```python
from build123d import *

# Parameters (mm, degrees)
SKETCH1_W           = 25
SKETCH1_H           = 0.7
BOSS_EXTRUDE1_DEPTH = 40
SKETCH2_R           = 2.15
SKETCH2_R_2         = 1.5
CUT_EXTRUDE1_DEPTH  = 40


with BuildPart() as part:
    # Sketch1 → Boss-Extrude1 (new body)
    with BuildSketch(Plane(origin=(0, 0, 0), x_dir=(1, 0, 0), z_dir=(0, 1, 0))):
        with Locations((12.5, 0.35)):
            Rectangle(SKETCH1_W, SKETCH1_H)
    extrude(amount=BOSS_EXTRUDE1_DEPTH)

    # Sketch2 → Cut-Extrude1 (cut)
    with BuildSketch(Plane.XY):
        with Locations((4, 35)):
            Circle(SKETCH2_R)
        with Locations((4, 25)):
            Circle(SKETCH2_R)
        with Locations((4, 15)):
            Circle(SKETCH2_R_2)
        with Locations((4, 5)):
            Circle(SKETCH2_R_2)
        with Locations((19, 15)):
            Circle(SKETCH2_R_2)
        with Locations((19, 5)):
            Circle(SKETCH2_R_2)
    extrude(amount=-CUT_EXTRUDE1_DEPTH, mode=Mode.SUBTRACT)


solid = part.part
```
Verification items for the finished model (mm, model axes). Round coordinates to 2 decimals unless told otherwise and drop trailing zeros. Write each loop counter-clockwise with the first axis right and the second up, starting at its lowest first coordinate (ties: lowest second). Pieces come first, ordered by that corner, then holes.
1. Section check C-C on x = 4. Enter the section's corners in (y, z), plus the area to 3 significant figures.
2. Gauge pin test, flat end, axial feed: P1, Ø1.8, axis at x = 4, y = 15, coming from the +Z side. Record the tip position at first contact, or that the pin passes through.
3. Draft check along X on faces 1 (the flat face through (12, 20, -0.7)), 2 (the cylindrical face through (2.294, 23.692, -0.345)). Enter one of: +X half, -X half, draft (parallel to the pull), parting line (faces both ways), or undercut.
4. Section check D-D on z = -0.45. Enter the section's corners in (x, y), plus the area to 3 significant figures.
5. Scan lines: L1, parallel to Y at x = 19, z = -0.3; L2, parallel to Y at x = 4, z = -0.5. Record each from-to range of solid material in increasing order.
6. Section check B-B on y = 15. Enter the section's corners in (x, z), plus the area to 3 significant figures.
7. Section check A-A on x = 19. Enter the section's corners in (y, z), plus the area to 3 significant figures.
Answer:
1. outline: (0, -0.7) - (3.5, -0.7) - (3.5, 0) - (0, 0) - close; (6.5, -0.7) - (13.5, -0.7) - (13.5, 0) - (6.5, 0) - close; (16.5, -0.7) - (22.85, -0.7) - (22.85, 0) - (16.5, 0) - close; (27.15, -0.7) - (32.85, -0.7) - (32.85, 0) - (27.15, 0) - close; (37.15, -0.7) - (40, -0.7) - (40, 0) - (37.15, 0) - close
1. area: 17.8 mm2
2. P1: passes through
3. face 1: draft
3. face 2: undercut
4. outline: (0, 0) - (25, 0) - (25, 40) - (0, 40) - close; hole circle Ø4.3 at (4, 25); hole circle Ø4.3 at (4, 35); hole circle Ø3 at (4, 5); hole circle Ø3 at (4, 15); hole circle Ø3 at (19, 5); hole circle Ø3 at (19, 15)
4. area: 943 mm2
5. L1: y = 0 to 3.5, 6.5 to 13.5, 16.5 to 40
5. L2: y = 0 to 3.5, 6.5 to 13.5, 16.5 to 22.85, 27.15 to 32.85, 37.15 to 40
6. outline: (0, -0.7) - (2.5, -0.7) - (2.5, 0) - (0, 0) - close; (5.5, -0.7) - (17.5, -0.7) - (17.5, 0) - (5.5, 0) - close; (20.5, -0.7) - (25, -0.7) - (25, 0) - (20.5, 0) - close
6. area: 13.3 mm2
7. outline: (0, -0.7) - (3.5, -0.7) - (3.5, 0) - (0, 0) - close; (6.5, -0.7) - (13.5, -0.7) - (13.5, 0) - (6.5, 0) - close; (16.5, -0.7) - (40, -0.7) - (40, 0) - (16.5, 0) - close
7. area: 23.8 mm2
